Source: three-view drawing plus pictorial views. Frame: mm from the lowest corner of the part. Give positions to 0.01 mm unless a question says otherwise; leave off trailing zeros. Write each loop counter-clockwise with the first axis right and the second up, starting at its lowest first coordinate (ties: lowest second). Pieces come first, ordered by that corner, then holes. Notation, with made-up numbers: (31, 46.5) -> (40, 46.5) arc R14 cw to (40, 65.5) -> close; hole circle Ø5 at (-16.5, 19.5). An arc over 180 degrees is marked (long way). Use a Markdown table: item, result. Add a question column.
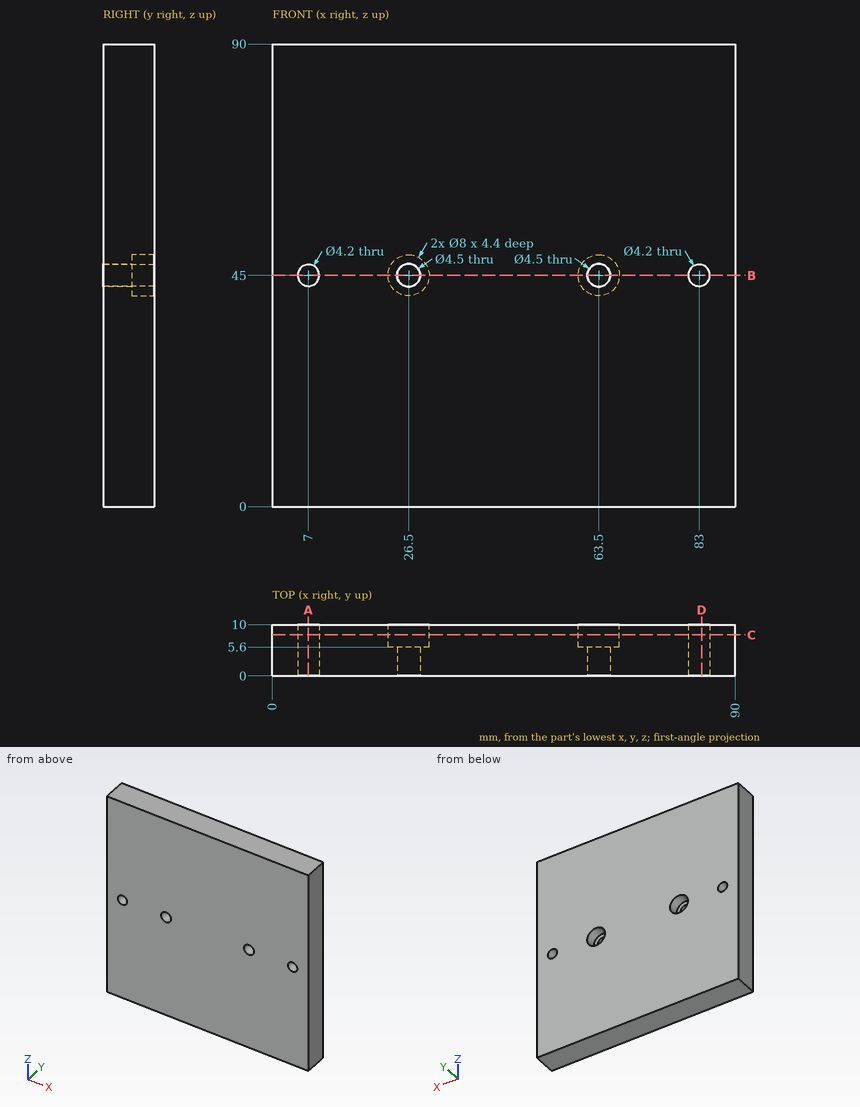
(1) First-contact query: pin 1 Ø4 at (x, z) = (65, 45.5) entering from +Y; pin 2 Ø4 at (x, y) = (33.5, 7.5) entering from -Z; pin 3 Ø3.5 at (x, z) = (63.5, 45) entering from +Y. Flat tips, straight axial feed; report the tip coordinate or a pass-through.
(2) Cut plane A-A on x = 7. Return the cut outline in (y, z), then the cut area to 3 significant figures.
(3) Cut plane B-B on z = 45. Return the cut outline in (x, y).
(4) Cut plane D-D on x = 83.5. Return the cut outline in (y, z), then the cut area to 3 significant figures.
(5) Cut plane C-C on y = 8. Return the cut outline in (x, z).
(6) Material intervals for L1, parallel to X at y = 8.25, z = 45; L2, parallel to X at y = 2.2, z = 45; L3, parallel to Z at x = 7, y = 7.25, sorted ascending.
Output:
| question | item | result |
|---|---|---|
| 1 | pin 1 | y = 5.6 |
| 1 | pin 2 | z = 0 |
| 1 | pin 3 | through |
| 2 | outline | (0, 0) -> (10, 0) -> (10, 42.9) -> (0, 42.9) -> close; (0, 47.1) -> (10, 47.1) -> (10, 90) -> (0, 90) -> close |
| 2 | area | 858 mm^2 |
| 3 | outline | (0, 0) -> (4.9, 0) -> (4.9, 10) -> (0, 10) -> close; (9.1, 0) -> (24.25, 0) -> (24.25, 5.6) -> (22.5, 5.6) -> (22.5, 10) -> (9.1, 10) -> close; (28.75, 0) -> (61.25, 0) -> (61.25, 5.6) -> (59.5, 5.6) -> (59.5, 10) -> (30.5, 10) -> (30.5, 5.6) -> (28.75, 5.6) -> close; (65.75, 0) -> (80.9, 0) -> (80.9, 10) -> (67.5, 10) -> (67.5, 5.6) -> (65.75, 5.6) -> close; (85.1, 0) -> (90, 0) -> (90, 10) -> (85.1, 10) -> close |
| 4 | outline | (0, 0) -> (10, 0) -> (10, 42.96) -> (0, 42.96) -> close; (0, 47.04) -> (10, 47.04) -> (10, 90) -> (0, 90) -> close |
| 4 | area | 859 mm^2 |
| 5 | outline | (0, 0) -> (90, 0) -> (90, 90) -> (0, 90) -> close; hole circle Ø4.2 at (7, 45); hole circle Ø8 at (26.5, 45); hole circle Ø8 at (63.5, 45); hole circle Ø4.2 at (83, 45) |
| 6 | L1 | 0 to 4.9, 9.1 to 22.5, 30.5 to 59.5, 67.5 to 80.9, 85.1 to 90 |
| 6 | L2 | 0 to 4.9, 9.1 to 24.25, 28.75 to 61.25, 65.75 to 80.9, 85.1 to 90 |
| 6 | L3 | 0 to 42.9, 47.1 to 90 |
